from build123d import *

# Parameters (mm, degrees)
F0_W     = 35
F0_H     = 32
F1_DEPTH = 1.5
F2_W     = 16
F2_H     = 20
F3_DEPTH = 12
F4_R     = 1.5
F5_DEPTH = 6
F6_W     = 1
F6_H     = 5
F7_DEPTH = 1.5


with BuildPart() as f1:
    # F0 (on Top) → F1 (new body)
    with BuildSketch(Plane.XY):
        Rectangle(F0_W, F0_H)
    extrude(amount=F1_DEPTH)

    # F2 (on face) → F3 (join)
    with BuildSketch(Plane.XY.offset(1.5)):
        with Locations((-0.5, 6)):
            Rectangle(F2_W, F2_H)
    extrude(amount=F3_DEPTH)

    # F4 (on face) → F5 (join)
    with BuildSketch(Plane.XY.offset(1.5)):
        with Locations((11.5, 9)):
            Circle(F4_R)
        with Locations((11.5, 4)):
            Circle(F4_R)
        with Locations((11.5, -1)):
            Circle(F4_R)
        with Locations((11.5, -6)):
            Circle(F4_R)
    extrude(amount=F5_DEPTH)

    # F6 (on face) → F7 (cut, through all)
    with BuildSketch(Plane.XY.offset(1.5)):
        with Locations((-14, 13.5)):
            Rectangle(F6_W, F6_H)
        with Locations((-14, 6.5)):
            Rectangle(F6_W, F6_H)
        with Locations((-14, -0.5)):
            Rectangle(F6_W, F6_H)
        with Locations((-14, -7.5)):
            Rectangle(F6_W, F6_H)
        with Locations((-14, -14.5)):
            Rectangle(F6_W, F6_H)
        with Locations((15, -13.5)):
            Rectangle(F6_W, F6_H)
        with Locations((15, -6.5)):
            Rectangle(F6_W, F6_H)
        with Locations((15, 0.5)):
            Rectangle(F6_W, F6_H)
        with Locations((15, 7.5)):
            Rectangle(F6_W, F6_H)
        with Locations((15, 14.5)):
            Rectangle(F6_W, F6_H)
    extrude(amount=-F7_DEPTH, mode=Mode.SUBTRACT)


solid = f1.part
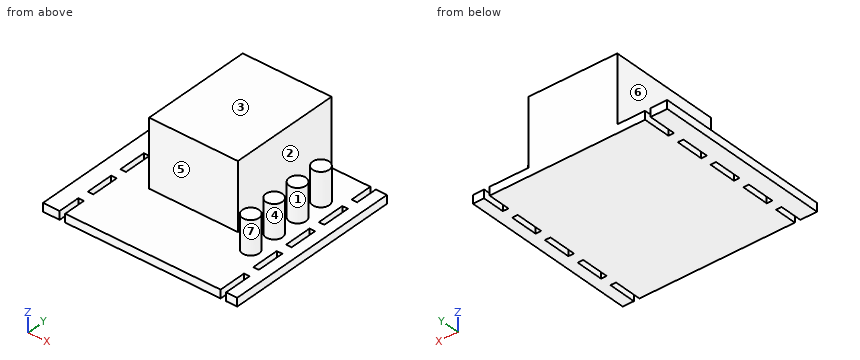
Work out the finished part from the listing and answer in its coordinate system (mm). Face numbers are marked on the shaded views. A direction names the side the tool comes from. Coordinates: 2 decimals unless noted, no trailing zeros. Write each loop counter-clockwise with the first axis right and the second up, starting at its lowest first coordinate (ties: lowest second). Pieces come first, ordered by that corner, then holes. Notation, with made-up numbers: M 65.5,-19.75 L 109.5,-19.75 A10 cw 109.5,-8.75 Z; hole C 36,-29.5 d5. An arc over 180 degrees is marked long. Answer as CSV lines item,"result". Start each with the question number.
Item 1: Section D-D on y = -12.5 is taken. Write down the section's boundary in (x, z).
Item 2: Determine the mould class of the marked faces 4, 5, 6 and 7 for opening direction X: released by +X, released by -X, zero draft, split by the parting line, or undercut.
Item 3: Flat-ended cylindrical pins translate along their axes: P1, Ø1.5, axis at x = 11.5, y = 8.5, coming from the +Z side; P2, Ø2, axis at x = 10.5, z = 8, coming from the +Y side; P3, Ø0.8, axis at x = 15, z = 0.5, coming from the +Y side; P4, Ø8, axis at x = 13, y = -1, coming from the -Z side. Find the tip coordinate at first contact, or state that the pin passes through.
Item 4: A tool of negligible diameter and unlimited length cuts with its end or side. For the marked faces 1, 2 and 3, from which of +Z, -Z, +X, -X, +Y, -Y can it reach the whole face along a straight path? Write none if from no direction.
Item 5: Section A-A on x = 15 is taken. Write down the section's boundary in (y, z), and give its area (3 significant figures).
Item 6: Consider L1, parallel to X at y = -13, z = 0.75; L2, parallel to Y at x = 12, z = 2.75; L3, parallel to Z at x = 9, y = -3. Determine where each line is inside the solid, lowest interval first.
Item 7: Section C-C on y = 14 is taken. Write down the section's boundary in (x, z).
Item 8: Section B-B on z = 2.5 is taken. Write down the section's boundary in (x, y), and give its area (3 significant figures).
Checks:
1,outline,"M -17.5,0 L -14.5,0 L -14.5,1.5 L -17.5,1.5 Z; M -13.5,0 L 14.5,0 L 14.5,1.5 L -13.5,1.5 Z; M 15.5,0 L 17.5,0 L 17.5,1.5 L 15.5,1.5 Z"
2,face 4,"undercut"
2,face 5,"zero draft"
2,face 6,"released by -X"
2,face 7,"split by the parting line"
3,P1,"stops at z = 7.5"
3,P2,"stops at y = 10.49"
3,P3,"stops at y = 12"
3,P4,"stops at z = 0"
4,face 1,"+Z"
4,face 2,"+Z, +Y, -Y"
4,face 3,"+Z, +X, -X, +Y, -Y"
5,outline,"M -11,0 L -9,0 L -9,1.5 L -11,1.5 Z; M -4,0 L -2,0 L -2,1.5 L -4,1.5 Z; M 3,0 L 5,0 L 5,1.5 L 3,1.5 Z; M 10,0 L 12,0 L 12,1.5 L 10,1.5 Z"
5,area,"12.0 mm²"
6,L1,"x = -17.5 to -14.5, -13.5 to 14.5, 15.5 to 17.5"
6,L2,"y = -7.41 to -4.59, -2.41 to 0.41, 2.59 to 5.41, 7.59 to 10.41"
6,L3,"z = 0 to 1.5"
7,outline,"M -17.5,0 L -14.5,0 L -14.5,1.5 L -17.5,1.5 Z; M -13.5,0 L 14.5,0 L 14.5,1.5 L 7.5,1.5 L 7.5,13.5 L -8.5,13.5 L -8.5,1.5 L -13.5,1.5 Z; M 15.5,0 L 17.5,0 L 17.5,1.5 L 15.5,1.5 Z"
8,outline,"M -8.5,-4 L 7.5,-4 L 7.5,16 L -8.5,16 Z; C 11.5,-6 d3; C 11.5,-1 d3; C 11.5,4 d3; C 11.5,9 d3"
8,area,"348 mm²"
